```python
from build123d import *

# Parameters (mm, degrees)
BOSS_EXTRUDE1_DEPTH      = 914.4
BOSS_EXTRUDE1_DEPTH_BACK = 914.4
FILLET1_R                = 1.905


with BuildPart() as part:
    # Sketch4 → Boss-Extrude1 (new body, two sides)
    with BuildSketch(Plane.XY) as boss_extrude1_sk:
        with BuildLine():
            Line((-7.9375, -6.0325), (-7.9375, 12.7))
            Line((-7.9375, 12.7), (-12.7, 12.7))
            Line((-12.7, 12.7), (-12.7, -12.7))
            Line((-12.7, -12.7), (12.7, -12.7))
            Line((12.7, -12.7), (12.7, -7.9375))
            Line((12.7, -7.9375), (-6.0325, -7.9375))
            ThreePointArc((-6.0325, -7.9375), (-7.379538418, -7.379538418), (-7.9375, -6.0325))
        make_face()
    extrude(amount=BOSS_EXTRUDE1_DEPTH)
    extrude(boss_extrude1_sk.sketch, amount=-BOSS_EXTRUDE1_DEPTH_BACK)

    # Fillet1
    fillet1_edges = [part.edges().sort_by_distance(p)[0] for p in [
        (-7.9375, 12.7, 0),
        (12.7, -7.9375, 0),
        (12.7, -12.7, 0),
        (-12.7, -12.7, 0),
        (-12.7, 12.7, 0),
    ]]
    fillet(fillet1_edges, radius=FILLET1_R)


solid = part.part
```
Here's how the part is built. I have some questions about the finished solid (model axes, mm). Give positions to 0.01 mm unless a question says otherwise; leave off trailing zeros. Loops run counter-clockwise (first coordinate to the right, second up) from the corner with the lowest first, then second, coordinate; pieces in that order, holes last. Notation, with made-up numbers: M -18.5,-25 L 39.5,-25 A18 ccw 39.5,0 Z; hole C 22,72 d5. An arc over 180 degrees is marked long. Return JSON: item names as keys, results as strings.
Item 1: Imagine slicing it at A-A on z = -588. List the corners of the cut face in (x, y) for me (1 decimal), then the cut area to 3 significant figures.
A:
{"outline": "M -12.7,-10.8 A1.9 ccw -10.8,-12.7 L 10.8,-12.7 A1.9 ccw 12.7,-10.8 L 12.7,-9.8 A1.9 ccw 10.8,-7.9 L -6,-7.9 A1.9 cw -7.9,-6 L -7.9,10.8 A1.9 ccw -9.8,12.7 L -10.8,12.7 A1.9 ccw -12.7,10.8 Z", "area": "216 mm^2"}
Item 2: Imagine slicing it at B-B on y = 5.5. List the corners of the cut face in (x, z) for me, then the cut area to 3 significant figures.
A:
{"outline": "M -12.7,-914.4 L -7.94,-914.4 L -7.94,914.4 L -12.7,914.4 Z", "area": "8,710 mm^2"}
Item 3: Please list where these lines run through material, in increasing order: line 1 (Y direction, x = -3.5, z = 731); line 2 (X direction, y = -9.5, z = 194.5).
A:
{"line 1": "y = -12.7 to -7.94", "line 2": "x = -12.7 to 12.67"}
Item 4: I'm going to push flat-ended pins straight in: pin 1 Ø8.5 at (x, z) = (4, 86) entering from +Y; pin 2 Ø8.5 at (y, z) = (2, 89) entering from +X. Where does each tip first touch, or does it pass through?
A:
{"pin 1": "stops at y = -7.94", "pin 2": "stops at x = -7.94"}
